from build123d import *

# Parameters (mm, degrees)
CUT_EXTRUDE_START        = -4
CUT_EXTRUDE_7_DEPTH      = 8
SKETCH_5_R               = 2.75
CUT_EXTRUDE_2_DEPTH      = 8
SKETCH_6_R               = 2.75
CUT_EXTRUDE_3_DEPTH      = 8
CUT_EXTRUDE_5_DEPTH      = 41.917600125
CUT_EXTRUDE_5_DEPTH_BACK = 41.917600125
SKETCH_8_R               = 5
EXTRUDE_START            = -75
SKETCH_10_R              = 5
EXTRUDE_1_DEPTH          = 150


with BuildPart() as part:
    # 草图3 → 旋转1 (revolve)
    with BuildSketch(Plane(origin=(0, 0, 0), x_dir=(0, 0, -1), z_dir=(1, 0, 0)), mode=Mode.PRIVATE) as revolve_1_sk:
        Polygon((-4, 0), (-4, 21), (4, 21), (4, 11), (31, 11), (31, 0), align=None)
    revolve(revolve_1_sk.sketch.rotate(Axis((0, 0, 4), (0, 0, -1)), 180), axis=Axis((0, 0, 4), (0, 0, -1)))

    # 草图13 → 切除-拉伸7 (cut)
    with BuildSketch(Plane.XY.offset(CUT_EXTRUDE_START)):
        with BuildLine():
            Line((-16.5, -12.990381057), (-16.5, 12.990381057))
            ThreePointArc((-16.5, 12.990381057), (-21, 0), (-16.5, -12.990381057))
        make_face()
        with BuildLine():
            Line((16.5, 12.990381057), (16.5, -12.990381057))
            ThreePointArc((16.5, -12.990381057), (21, 0), (16.5, 12.990381057))
        make_face()
    extrude(amount=CUT_EXTRUDE_7_DEPTH, mode=Mode.SUBTRACT)

    # 草图5 → 切除-拉伸2 (cut)
    with BuildSketch(Plane.XY.offset(CUT_EXTRUDE_START)):
        with Locations((-11.313708499, 11.313708499)):
            Circle(SKETCH_5_R)
        with Locations((11.313708499, 11.313708499)):
            Circle(SKETCH_5_R)
    cut_extrude_2 = extrude(amount=CUT_EXTRUDE_2_DEPTH, mode=Mode.SUBTRACT)

    # 镜向1: 切除-拉伸2 across plane
    add(cut_extrude_2.mirror(Plane.ZX), mode=Mode.SUBTRACT)

    # 草图6 → 切除-拉伸3 (cut)
    with BuildSketch(Plane.XY.offset(CUT_EXTRUDE_START)):
        with Locations((0, 16)):
            Circle(SKETCH_6_R)
    cut_extrude_3 = extrude(amount=CUT_EXTRUDE_3_DEPTH, mode=Mode.SUBTRACT)

    # 镜向2: 切除-拉伸3 across plane
    add(cut_extrude_3.mirror(Plane.ZX), mode=Mode.SUBTRACT)

    # 草图8 → 切除-拉伸5 (cut, two sides: drawn at the far end of the back side and taken through both)
    with BuildSketch(Plane.XY.offset(-CUT_EXTRUDE_5_DEPTH_BACK)):
        Circle(SKETCH_8_R)
    extrude(amount=CUT_EXTRUDE_5_DEPTH + CUT_EXTRUDE_5_DEPTH_BACK, mode=Mode.SUBTRACT)


with BuildPart() as body_2:
    # 草图10 → 凸台-拉伸1 (new body)
    with BuildSketch(Plane.XY.offset(EXTRUDE_START)):
        Circle(SKETCH_10_R)
    extrude(amount=EXTRUDE_1_DEPTH)


solid = part.part
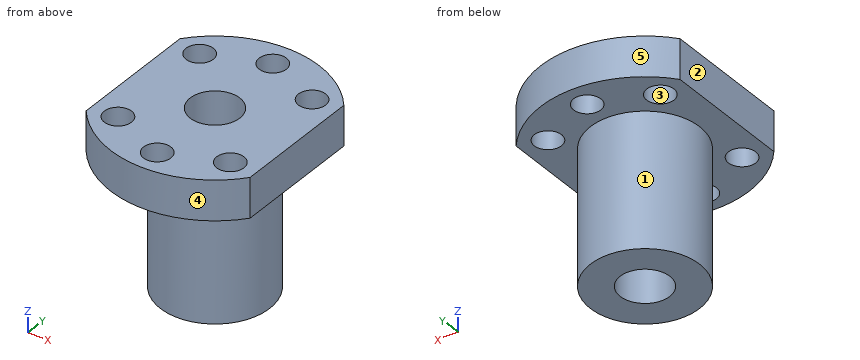
Read the model definition and answer for the solid it produces. Units are mm, in the model's axes. Face numbers are marked on the shaded views. A direction names the side the tool comes from. Give positions to 0.01 mm unless a question says otherwise; leave off trailing zeros. Loops run counter-clockwise (first coordinate to the right, second up) from the corner with the lowest first, then second, coordinate; pieces in that order, holes last. Notation, with made-up numbers: (54, 86) -> (102, 86) arc R25 ccw to (102, 123) -> close; hole circle Ø1 at (35.25, 14.5). An arc over 180 degrees is marked (long way). Answer as CSV lines item,"result".
Item 1: Find section D-D on z = -15.5. Give the vertices of the cut face in (x, y), plus the area to 3 significant figures.
Returned:
outline,"circle Ø22 at (0, 0); hole circle Ø10 at (0, 0)"
area,"302 mm²"
Item 2: Find section B-B on y = 0. Give the vertices of the cut face in (x, z), plus the area to 3 significant figures.
Returned:
outline,"(-16.5, -4) -> (-11, -4) -> (-11, -31) -> (-5, -31) -> (-5, 4) -> (-16.5, 4) -> close; (5, -31) -> (11, -31) -> (11, -4) -> (16.5, -4) -> (16.5, 4) -> (5, 4) -> close"
area,"508 mm²"
Item 3: Find section A-A on x = 0. Give the vertices of the cut face in (y, z).
Returned:
outline,"(-21, -4) -> (-18.75, -4) -> (-18.75, 4) -> (-21, 4) -> close; (-13.25, -4) -> (-11, -4) -> (-11, -31) -> (-5, -31) -> (-5, 4) -> (-13.25, 4) -> close; (5, -31) -> (11, -31) -> (11, -4) -> (13.25, -4) -> (13.25, 4) -> (5, 4) -> close; (18.75, -4) -> (21, -4) -> (21, 4) -> (18.75, 4) -> close"
Item 4: Each of these flat-tipped pins is pushed along its axis until it touches: pin 1 (6.5 mm diameter, centred on x = 0, y = -16, fed in from -Z); pin 2 (10 mm diameter, centred on x = -3.5, z = -26.5, fed in from +Y); pin 3 (2 mm diameter, centred on x = -4.5, z = -16, fed in from +Y). Where does it stop, or does it pass through?
Returned:
pin 1,"stops at z = -4"
pin 2,"stops at y = 11"
pin 3,"stops at y = 10.43"
Item 5: Determine the mould class of the marked faces 3, 4 and 5 for opening direction Y: +Y half, -Y half, draft (parallel to the pull), parting line (faces both ways), or undercut.
Returned:
face 3,"undercut"
face 4,"-Y half"
face 5,"+Y half"
Item 6: For the marked faces 1 and 2, determine the directions among +Z, -Z, +X, -X, +Y, -Y from which every point of the face is accessible in a straight line to the end or side of a thin tool.
Returned:
face 1,"-Z"
face 2,"+Z, -Z, -X, +Y, -Y"
Item 7: Consider line 1 (Y direction, x = 0, z = 2); line 2 (X direction, y = 0, z = -7); line 3 (Z direction, x = -11, y = -15). Determine where each line is inside the solid, lowest interval first. Write a range as [from, to].
Returned:
line 1,"y = [-21, -18.75], [-13.25, -5], [5, 13.25], [18.75, 21]"
line 2,"x = [-11, -5], [5, 11]"
line 3,"z = [-4, 4]"
Item 8: Find section C-C on x = 12. Give the vertices of the cut face in (y, z).
Returned:
outline,"(-17.23, -4) -> (-13.98, -4) -> (-13.98, 4) -> (-17.23, 4) -> close; (-8.65, -4) -> (8.65, -4) -> (8.65, 4) -> (-8.65, 4) -> close; (13.98, -4) -> (17.23, -4) -> (17.23, 4) -> (13.98, 4) -> close"
